Can you work these out from the drawing? Everything is in mm from the part's minimum corner. Round coordinates to 2 decimals unless told otherwise and drop trailing zeros. Loops run counter-clockwise (first coordinate to the right, second up) from the corner with the lowest first, then second, coordinate; pieces in that order, holes last. Notation, with made-up numbers: M 64,-4.75 L 98,-4.75 A37 cw 98,32.25 Z; hole C 44,-39 d5. An arc over 180 degrees is marked long. Use a Markdown table: item, result.
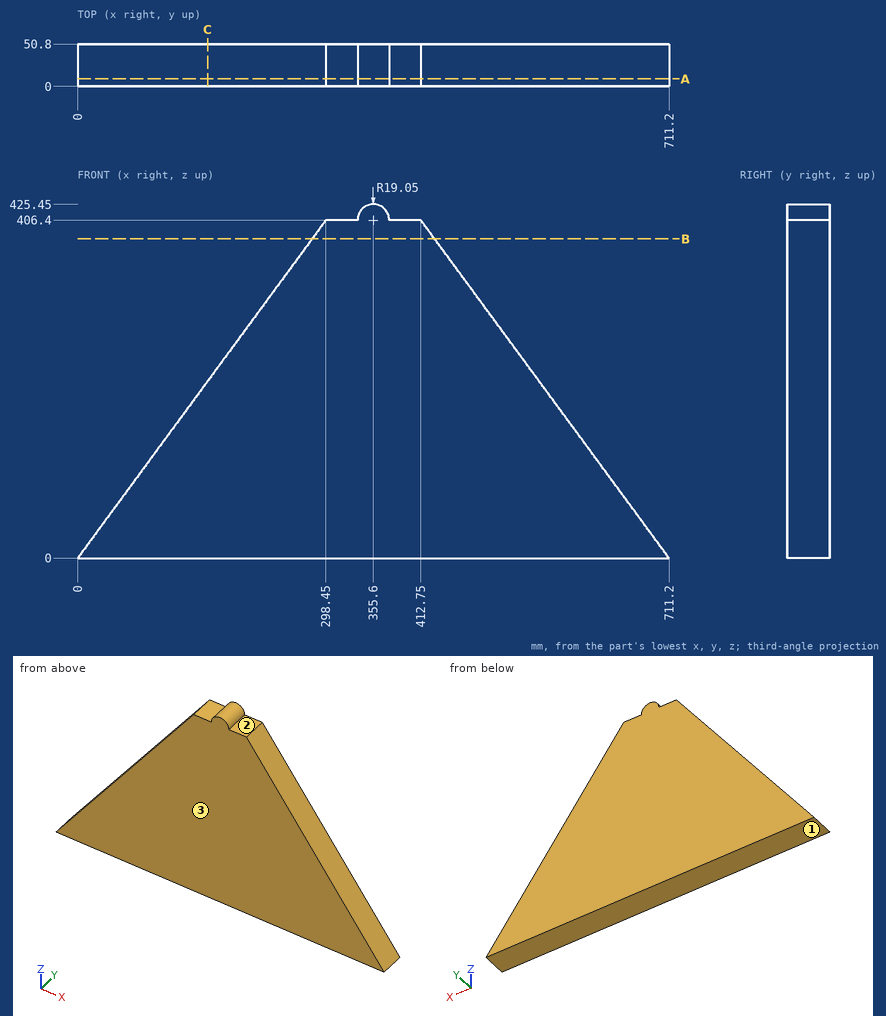
1. Imagine slicing it at B-B, the plane z = 384. Write out the boundary of the cut face in (x, y).
Answer sheet:
| item | result |
|---|---|
| outline | M 282,0 L 429.2,0 L 429.2,50.8 L 282,50.8 Z |
2. For pin 1 Ø4 at (x, z) = (403.5, 161.5) entering from -Y; pin 2 Ø4 at (x, y) = (432, 44.5) entering from +Z; pin 3 Ø4 at (y, z) = (31.5, 268.5) entering from -X; pin 4 Ø12 at (x, y) = (90.5, 24) entering from +Z, each with a flat end and sliding along its axis, tell me the tip position at first contact or that it passes through.
Answer sheet:
| item | result |
|---|---|
| pin 1 | y = 0 |
| pin 2 | z = 382.91 |
| pin 3 | x = 195.71 |
| pin 4 | z = 131.4 |
3. I need wall thicknesses on probe 1 along Z at (x, y) = (315.5, 31.5); probe 2 along X at (y, z) = (40, 135.5); probe 3 along Z at (x, y) = (245, 34). Which ranges of each line are inside material? Lowest first, please. Write a range as from..to.
Answer sheet:
| item | result |
|---|---|
| probe 1 | 0..406.4 |
| probe 2 | 99.51..611.69 |
| probe 3 | 0..333.62 |
4. We'd pull the mould along Z, two halves only. Please class the marked faces 1, 2 and 3: +Z half, -Z half, draft (parallel to the pull), parting line (faces both ways), or undercut.
Answer sheet:
| item | result |
|---|---|
| face 1 | -Z half |
| face 2 | +Z half |
| face 3 | draft |
5. Imagine slicing it at A-A, the plane y = 9. Write out the boundary of the cut face in (x, z), then the cut area to 3 significant figures.
Answer sheet:
| item | result |
|---|---|
| outline | M 0,0 L 711.2,0 L 412.75,406.4 L 374.65,406.4 A19.05 ccw 336.55,406.4 L 298.45,406.4 Z |
| area | 168,000 mm2 |
6. Imagine slicing it at C-C, the plane x = 156.5. Write out the boundary of the cut face in (y, z).
Answer sheet:
| item | result |
|---|---|
| outline | M 0,0 L 50.8,0 L 50.8,213.11 L 0,213.11 Z |
